from build123d import *

# Parameters (mm, degrees)
BOSS_EXTRUDE1_DEPTH = 5


with BuildPart() as part:
    # Sketch1 → Boss-Extrude1 (new body)
    with BuildSketch(Plane(origin=(0, 0, 0), x_dir=(0, 0, -1), z_dir=(1, 0, 0))):
        with BuildLine():
            Line((-11, 0), (-11, 20))
            Line((-11, 20), (11, 20))
            Line((11, 20), (11, 0))
            ThreePointArc((11, 0), (0, -11), (-11, 0))
        make_face()
        with BuildLine():
            Line((-2.5, 10), (2.5, 10))
            Line((2.5, 10), (2.5, 7.599342077))
            ThreePointArc((2.5, 7.599342077), (0, -8), (-2.5, 7.599342077))
            Line((-2.5, 7.599342077), (-2.5, 10))
        make_face(mode=Mode.SUBTRACT)
    extrude(amount=BOSS_EXTRUDE1_DEPTH)


solid = part.part
Work out the finished part from the listing and answer in its coordinate system (mm). A direction names the side the tool comes from. Give positions to 0.01 mm unless a question says otherwise; leave off trailing zeros. Order: outer loops, then holes, each group sorted by start corner. A loop starts at its lowest first (then second) coordinate and runs counter-clockwise, first axis right, second up. Notation, with made-up numbers: (35.25, 50.5) - (85.25, 50.5) arc R24 cw to (85.25, 75.5) - close; hole circle Ø8 at (1, -1). An arc over 180 degrees is marked (long way). Answer as CSV lines item,"result". Start each with the question number.
Q1. For faces 1 (the face through (2, 9, -2.5)), 2 (the face through (5, 8, -3)), determine the directions among +Z, -Z, +X, -X, +Y, -Y from which every point of the face is accessible in a straight line to the end or side of a thin tool.
Q2. Given pin 1 Ø2 at (x, z) = (1, 2) entering from -Y, flat-ended and moving along its own axis, determine where the tip first touches the part or whether it passes through.
Q3. The part is cut by section A-A (z = 0). Write down the section's boundary in (x, y).
Q4. The part is cut by section B-B (y = -1.5). Write down the section's boundary in (x, z).
Q5. The part is cut by section C-C (x = 3). Write down the section's boundary in (y, z).
Q6. Find the intervals of material crossed by L1, parallel to Y at x = 1.4, z = 0; L2, parallel to Y at x = 0.65, z = 3; L3, parallel to Z at x = 0.65, y = -5 (3 decimals), in increasing order. Write a range as [from, to].
Q7. The part is cut by section D-D (z = 8.75). Write down the section's boundary in (x, y), then the cut area to 3 significant figures.
Check result:
1,face 1,"+X, -X"
1,face 2,"+Z, -Z, +X, +Y, -Y"
2,pin 1,"stops at y = -10.95"
3,outline,"(0, -11) - (5, -11) - (5, -8) - (0, -8) - close; (0, 10) - (5, 10) - (5, 20) - (0, 20) - close"
4,outline,"(0, -10.9) - (5, -10.9) - (5, -7.86) - (0, -7.86) - close; (0, 7.86) - (5, 7.86) - (5, 10.9) - (0, 10.9) - close"
5,outline,"(0, -11) - (20, -11) - (20, 11) - (0, 11) arc R11 ccw to start; hole (7.6, -2.5) - (10, -2.5) - (10, 2.5) - (7.6, 2.5) arc R8 ccw (long way) to start"
6,L1,"y = [-11, -8], [10, 20]"
6,L2,"y = [-10.58, -7.42], [7.42, 20]"
6,L3,"z = [-9.798, -6.245], [6.245, 9.798]"
7,outline,"(0, -6.67) - (5, -6.67) - (5, 20) - (0, 20) - close"
7,area,"133 mm²"
